```python
from build123d import *

# Parameters (mm, degrees)
F0_W     = 139.7
F0_H     = 101.6
F1_DEPTH = 1.5875
F2_R     = 2.413
F3_DEPTH = 25.4


with BuildPart() as f1:
    # F0 (on Top) → F1 (new body, symmetric)
    with BuildSketch(Plane.XY):
        Rectangle(F0_W, F0_H)
    extrude(amount=F1_DEPTH, both=True)

    # F2 (on face) → F3 (cut)
    with BuildSketch(Plane.XY.offset(1.5875)):
        with BuildLine():
            Line((63.5, -25.4), (65.913, -25.4))
            ThreePointArc((65.913, -25.4), (63.5, -22.987), (61.087, -25.4))
            Line((61.087, -25.4), (63.5, -25.4))
        make_face()
        with BuildLine():
            ThreePointArc((-65.913, -25.4), (-63.5, -27.813), (-61.087, -25.4))
            Line((-61.087, -25.4), (-65.913, -25.4))
        make_face()
        with BuildLine():
            Line((-65.913, -25.4), (-61.087, -25.4))
            ThreePointArc((-61.087, -25.4), (-63.5, -22.987), (-65.913, -25.4))
        make_face()
        with BuildLine():
            ThreePointArc((61.087, -25.4), (63.5, -27.813), (65.913, -25.4))
            Line((65.913, -25.4), (63.5, -25.4))
            Line((63.5, -25.4), (61.087, -25.4))
        make_face()
        with BuildLine():
            ThreePointArc((63.5, 21.463), (61.793751337, 17.343751337), (65.913, 19.05))
            ThreePointArc((65.913, 19.05), (65.206248663, 20.756248663), (63.5, 21.463))
        make_face()
        with Locations((19.05, 44.45)):
            Circle(F2_R)
        with BuildLine():
            ThreePointArc((-19.05, 46.863), (-20.756248663, 42.743751337), (-16.637, 44.45))
            ThreePointArc((-16.637, 44.45), (-17.343751337, 46.156248663), (-19.05, 46.863))
        make_face()
        with Locations((-63.5, 19.05)):
            Circle(F2_R)
        with Locations((-31.75, -41.402)):
            Circle(F2_R)
        with Locations((31.75, -41.402)):
            Circle(F2_R)
    extrude(amount=-F3_DEPTH, mode=Mode.SUBTRACT)


solid = f1.part
```
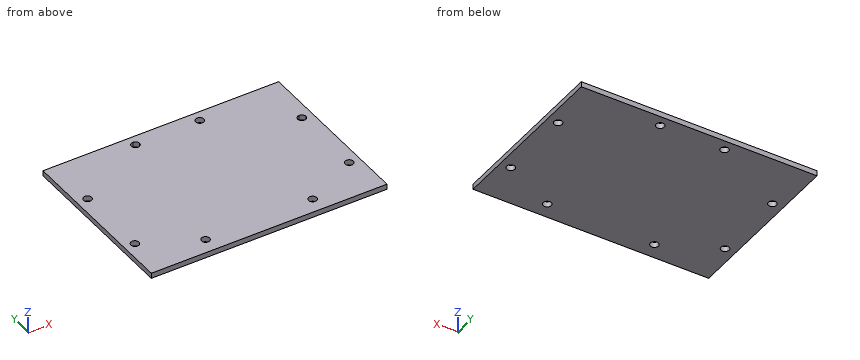
Read the model definition and answer for the solid it produces. Units are mm, in the model's axes. Round coordinates to 2 decimals unless told otherwise and drop trailing zeros. Write each loop counter-clockwise with the first axis right and the second up, starting at its lowest first coordinate (ties: lowest second). Pieces come first, ordered by that corner, then holes. Notation, with made-up numbers: (-4, -22.75) - (33, -22.75) arc R24 cw to (33, 14.25) - close; hole circle Ø6 at (59, 41). An arc over 180 degrees is marked (long way). Use CSV: the item, a comma, the result in double quotes.
Q1. Each of these flat-tipped pins is pushed along its axis until it touches: pin 1 Ø6.5 at (x, y) = (-31.75, -41.402) entering from +Z; pin 2 Ø4.5 at (x, y) = (63.5, 19.05) entering from -Z. Where does it stop, or does it pass through?
Values:
pin 1,"stops at z = 1.59"
pin 2,"passes through"
Q2. Straight lines are drawn through the part: line 1 along Y through (x, z) = (63.5, 0.05); line 2 along X through (y, z) = (-25.5, -1.5); line 3 along Y through (x, z) = (-19.05, 0.9). For each, find the intervals that lie inside material, in ascending order.
Values:
line 1,"y = -50.8 to -27.81, -22.99 to 16.64, 21.46 to 50.8"
line 2,"x = -69.85 to -65.91, -61.09 to 61.09, 65.91 to 69.85"
line 3,"y = -50.8 to 42.04, 46.86 to 50.8"
Q3. Find section A-A, the plane y = -25.4. Write down the section's boundary in (x, z), then the cut area to 3 significant figures.
Values:
outline,"(-69.85, -1.59) - (-65.91, -1.59) - (-65.91, 1.59) - (-69.85, 1.59) - close; (-61.09, -1.59) - (61.09, -1.59) - (61.09, 1.59) - (-61.09, 1.59) - close; (65.91, -1.59) - (69.85, -1.59) - (69.85, 1.59) - (65.91, 1.59) - close"
area,"413 mm²"
Q4. Find section B-B, the plane x = 19.05. Write down the section's boundary in (y, z).
Values:
outline,"(-50.8, -1.59) - (42.04, -1.59) - (42.04, 1.59) - (-50.8, 1.59) - close; (46.86, -1.59) - (50.8, -1.59) - (50.8, 1.59) - (46.86, 1.59) - close"
